Build history of the part. All positions in model axes, mm. A direction names the side the tool comes from. Coordinates: 2 decimals unless noted, no trailing zeros. Order: outer loops, then holes, each group sorted by start corner. A loop starts at its lowest first (then second) coordinate and runs counter-clockwise, first axis right, second up. Notation, with made-up numbers: (77, 17.25) - (93, 17.25) arc R18 ccw to (93, 51.25) - close; hole circle Ø2 at (29.5, 71). An arc over 180 degrees is marked (long way). Answer as CSV lines item,"result". Start each with the question number.
from build123d import *

# Parameters (mm, degrees)
SKETCH1_R                        = 140
SKETCH1_R_2                      = 62.5
BOSS_EXTRUDE1_DEPTH              = 5
SKETCH1_3_R                      = 62.5
SKETCH1_3_R_2                    = 57.5
SKETCH1_3_R_3                    = 55
BOSS_EXTRUDE2_DEPTH              = 100
SKETCH1_4_R                      = 57.5
SKETCH1_4_R_2                    = 55
CUT_EXTRUDE1_DEPTH               = 20
CUT_EXTRUDE2_START               = -20
SKETCH2_R                        = 57.5
CUT_EXTRUDE2_DEPTH               = 20
F_10_0MM_DOWEL_HOLE1_D           = 10
F_10_0MM_DOWEL_HOLE1_CSINK_D     = 10.05
F_10_0MM_DOWEL_HOLE1_CSINK_ANGLE = 90
CUT_EXTRUDE3_DEPTH               = 5
RIB4_START                       = -2.5
RIB4_DEPTH                       = 5
RIB5_REACH                       = 223.811
SKETCH9_WALL_W                   = 565.734948258
SKETCH9_WALL_H                   = 5
RIB6_REACH                       = 223.811
SKETCH10_WALL_W                  = 565.734948258
SKETCH10_WALL_H                  = 5
RIB7_REACH                       = 223.811
SKETCH11_WALL_W                  = 565.734948258
SKETCH11_WALL_H                  = 5


# Read off the part's stored shape, not the designer's step: Rib4
with BuildPart() as part:
    # Sketch1 → Boss-Extrude1 (new body)
    with BuildSketch(Plane(origin=(0, 0, 0), x_dir=(1, 0, 0), z_dir=(0, 1, 0))):
        with Locations(Location((0, 0, 0), (0, 0, 270))):
            Circle(SKETCH1_R)
        with Locations(Location((0, 0, 0), (0, 0, 270))):
            Circle(SKETCH1_R_2, mode=Mode.SUBTRACT)
    extrude(amount=BOSS_EXTRUDE1_DEPTH)

    # Sketch1<3> → Boss-Extrude2 (add)
    # profile 1 of 2: a face of its own
    with BuildSketch(Plane(origin=(0, 0, 0), x_dir=(1, 0, 0), z_dir=(0, 1, 0))):
        with Locations(Location((0, 0, 0), (0, 0, 270))):
            Circle(SKETCH1_3_R)
        Circle(SKETCH1_3_R_2, mode=Mode.SUBTRACT)
    # profile 2 of 2: a face of its own
    with BuildSketch(Plane(origin=(0, 0, 0), x_dir=(1, 0, 0), z_dir=(0, 1, 0))):
        Circle(SKETCH1_3_R_2)
        with Locations(Location((0, 0, 0), (0, 0, 270))):
            Circle(SKETCH1_3_R_3, mode=Mode.SUBTRACT)
    extrude(amount=BOSS_EXTRUDE2_DEPTH)

    # Sketch1<4> → Cut-Extrude1 (cut)
    with BuildSketch(Plane(origin=(0, 0, 0), x_dir=(1, 0, 0), z_dir=(0, 1, 0))):
        with Locations(Location((0, 0, 0), (0, 0, 270))):
            Circle(SKETCH1_4_R)
        with Locations(Location((0, 0, 0), (0, 0, 270))):
            Circle(SKETCH1_4_R_2, mode=Mode.SUBTRACT)
    extrude(amount=CUT_EXTRUDE1_DEPTH, mode=Mode.SUBTRACT)

    # Sketch2 → Cut-Extrude2 (cut)
    with BuildSketch(Plane(origin=(0, 100, 0), x_dir=(1, 0, 0), z_dir=(0, 1, 0)).offset(CUT_EXTRUDE2_START)):
        with Locations(Location((0, 0, 0), (0, 0, 270))):
            Circle(SKETCH2_R)
    extrude(amount=CUT_EXTRUDE2_DEPTH, mode=Mode.SUBTRACT)

    # Ø10.0mm Dowel Hole1 (through all)
    with Locations(Plane.XZ):
        with Locations((-63.639461911, -63.639758703), (63.639461911, -63.639758703), (63.639461911, 63.639758703), (-63.639461911, 63.639758703), (-63.582280459, -63.582280459)):
            CounterSinkHole(F_10_0MM_DOWEL_HOLE1_D / 2, F_10_0MM_DOWEL_HOLE1_CSINK_D / 2, counter_sink_angle=F_10_0MM_DOWEL_HOLE1_CSINK_ANGLE)

    # Sketch8 → Cut-Extrude3 (cut)
    with BuildSketch(Plane(origin=(0, 0, 0), x_dir=(1, 0, 0), z_dir=(0, 1, 0))):
        with BuildLine():
            ThreePointArc((31.996881471, 136.294532451), (136.294532451, 136.294532451), (136.294532451, 31.996881471))
            Line((136.294532451, 31.996881471), (31.996881471, 136.294532451))
        make_face()
        with BuildLine():
            Line((31.996881471, -136.294532451), (136.294532451, -31.996881471))
            ThreePointArc((136.294532451, -31.996881471), (136.294532451, -136.294532451), (31.996881471, -136.294532451))
        make_face()
        with BuildLine():
            Line((-31.996881471, -136.294532451), (-84.145706961, -84.145706961))
            Line((-84.145706961, -84.145706961), (-136.294532451, -31.996881471))
            ThreePointArc((-136.294532451, -31.996881471), (-136.294532451, -136.294532451), (-31.996881471, -136.294532451))
        make_face()
        with BuildLine():
            Line((-136.294532451, 31.996881471), (-31.996881471, 136.294532451))
            ThreePointArc((-31.996881471, 136.294532451), (-136.294532451, 136.294532451), (-136.294532451, 31.996881471))
        make_face()
    extrude(amount=CUT_EXTRUDE3_DEPTH, mode=Mode.SUBTRACT)

    # Rib4 outline → Rib4 (add)
    with BuildSketch(Plane.XY.offset(RIB4_START)):
        Polygon((-61.5, 100), (-62.449979984, 98.772134715), (-135, 5), (-61, 5), (-61, 100), align=None)
    extrude(amount=RIB4_DEPTH)

    # Sketch9 wall → Rib5 (add, up to next)
    with BuildSketch(Plane(origin=(98.25, 52.5, 0), x_dir=(0.611921285633, -0.790918668505, 0), z_dir=(0.790918668505, 0.611921285633, 0)), mode=Mode.PRIVATE) as rib5_sk1:
        Rectangle(SKETCH9_WALL_W, SKETCH9_WALL_H)
    rib5_tool1 = extrude(rib5_sk1.sketch, amount=-RIB5_REACH, mode=Mode.PRIVATE) - part.part
    add(rib5_tool1.solids().sort_by_distance((98.25, 52.5, 0))[0])

    # Sketch10 wall → Rib6 (add, up to next)
    with BuildSketch(Plane(origin=(0, 52.5, 98.25), x_dir=(0, -0.790918668505, 0.611921285633), z_dir=(0, -0.611921285633, -0.790918668505)), mode=Mode.PRIVATE) as rib6_sk1:
        Rectangle(SKETCH10_WALL_W, SKETCH10_WALL_H)
    rib6_tool1 = extrude(rib6_sk1.sketch, amount=RIB6_REACH, mode=Mode.PRIVATE) - part.part
    add(rib6_tool1.solids().sort_by_distance((0, 52.5, 98.25))[0])

    # Sketch11 wall → Rib7 (add, up to next)
    with BuildSketch(Plane(origin=(0, 52.5, -98.25), x_dir=(0, -0.790918668505, -0.611921285633), z_dir=(0, 0.611921285633, -0.790918668505)), mode=Mode.PRIVATE) as rib7_sk1:
        Rectangle(SKETCH11_WALL_W, SKETCH11_WALL_H)
    rib7_tool1 = extrude(rib7_sk1.sketch, amount=-RIB7_REACH, mode=Mode.PRIVATE) - part.part
    add(rib7_tool1.solids().sort_by_distance((0, 52.5, -98.25))[0])


solid = part.part
(1) Pull direction X, two halves, no side cores. Call faces 5 (the flat face through (-83.416, 2.465, 84.876)), 6 (the flat face through (2.5, 39, -81)), 7 (the flat face through (-30, 80, 47)): +X half, -X half, draft (parallel to the pull), parting line (faces both ways), or undercut.
(2) Band-saw the part on B-B on z = -13. List the corners of the cut face in (x, y), plus the area to 3 significant figures.
(3) Band-saw the part on A-A on x = -9. List the corners of the cut face in (y, z), plus the area to 3 significant figures.
(4) Band-saw the part on C-C on y = 72. List the corners of the cut face in (x, z).
(5) Drop flat-ended pins along their axis: pin 1 Ø22 at (x, y) = (82.5, 54.5) entering from -Z; pin 2 Ø1.5 at (y, z) = (82, 50) entering from -X; pin 3 Ø12 at (x, z) = (-41, -71) entering from +Y. Give the stop position or say it passes through.
(6) Which spindle directions (+Z, -Z, +X, -X, +Y, -Y) get a long thin tool onto all of the face, cutting with end or side? Do faces 1 (the flat face through (-83, 32, 2.5)), 2 (the cylindrical face through (-56.133, 9.86, -12.465)), 3 (the flat face through (-2.5, 39, -81)), 4 (the flat face through (-0.04, 52.54, -98.22)). Say none if no direction does.
(7) Probe L1, parallel to Y at x = -77, z = 42.5; L2, parallel to X at y = 43.5, z = -95; L3, parallel to Z at x = -19, y = 8.5. List the from-to ranges inside material, lowest first. Write a range as [from, to].
(8) Band-saw the part on D-D on x = -118. List the corners of the cut face in (y, z).
Filled in:
1,face 5,"-X half"
1,face 6,"+X half"
1,face 7,"undercut"
2,outline,"(-139.4, 0) - (-56.01, 0) - (-56.01, 20) - (-53.44, 20) - (-53.44, 80) - (-56.01, 80) - (-56.01, 100) - (-61.13, 100) - (-61.13, 5) - (-139.4, 5) - close; (53.44, 20) - (56.01, 20) - (56.01, 0) - (139.4, 0) - (139.4, 5) - (61.13, 5) - (61.13, 100) - (56.01, 100) - (56.01, 80) - (53.44, 80) - close"
2,area,"2,120 mm^2"
3,outline,"(0, -139.71) - (5, -139.71) - (5, -61.85) - (100, -61.85) - (100, -56.79) - (80, -56.79) - (80, -54.26) - (20, -54.26) - (20, -56.79) - (0, -56.79) - close; (0, 56.79) - (20, 56.79) - (20, 54.26) - (80, 54.26) - (80, 56.79) - (100, 56.79) - (100, 61.85) - (5, 61.85) - (5, 139.71) - (0, 139.71) - close"
3,area,"2,090 mm^2"
4,outline,"(-83.16, -2.5) - (-62.45, -2.5) arc R62.5 ccw to (-2.5, -62.45) - (-2.5, -83.16) - (2.5, -83.16) - (2.5, -62.45) arc R62.5 ccw to (62.45, -2.5) - (83.16, -2.5) - (83.16, 2.5) - (62.45, 2.5) arc R62.5 ccw to (2.5, 62.45) - (2.5, 83.16) - (-2.5, 83.16) - (-2.5, 62.45) arc R62.5 ccw to (-62.45, 2.5) - (-83.16, 2.5) - close; hole circle Ø110 at (0, 0)"
5,pin 1,"stops at z = -2.5"
5,pin 2,"stops at x = -38.48"
5,pin 3,"stops at y = 5"
6,face 1,"+Z, -X, +Y"
6,face 2,"-Y"
6,face 3,"-Z, -X, +Y"
6,face 4,"-Z, +X, -X, +Y"
7,L1,"y = [0, 5]"
7,L2,"x = [-2.5, 2.5]"
7,L3,"z = [-59.54, -54.27], [54.27, 59.54]"
8,outline,"(0, -50.29) - (5, -50.29) - (5, -2.5) - (26.97, -2.5) - (26.97, 2.5) - (5, 2.5) - (5, 50.29) - (0, 50.29) - close"
